from build123d import *

# Parameters (mm, degrees)
SKETCH1_R           = 1.3
SKETCH1_R_2         = 0.3
BOSS_EXTRUDE1_DEPTH = 1
SKETCH1_3_R         = 0.7625
BOSS_EXTRUDE2_DEPTH = 0.7
BOSS_EXTRUDE3_DEPTH = 0.6
BOSS_EXTRUDE4_DEPTH = 0.6
BOSS_EXTRUDE5_DEPTH = 0.2
SKETCH5_R           = 0.3
BOSS_EXTRUDE6_DEPTH = 0.2


with BuildPart() as part:
    # Sketch1 → Boss-Extrude1 (new, symmetric)
    with BuildSketch(Plane.XY):
        Circle(SKETCH1_R)
        Circle(SKETCH1_R_2, mode=Mode.SUBTRACT)
    extrude(amount=BOSS_EXTRUDE1_DEPTH, both=True)



with BuildPart() as body_2:
    # Sketch1_3 → Boss-Extrude2 (new, symmetric)
    with BuildSketch(Plane.XY):
        with Locations((3.98, -0.68)):
            Circle(SKETCH1_3_R)
    extrude(amount=BOSS_EXTRUDE2_DEPTH, both=True)


with BuildPart() as part_1:
    add(part.part)

    add(body_2.part)  # Boss-Extrude3 merges body 2
    # Sketch1_4 → Boss-Extrude3 (add, symmetric)
    with BuildSketch(Plane.XY):
        with BuildLine():
            ThreePointArc((3.432931907, -1.211152286), (3.227898468, -0.554502849), (3.635027175, 0))
            Line((3.635027175, 0), (1.875255399, 0.852756227))
            Line((1.875255399, 0.852756227), (0.329330809, 1.257593423))
            ThreePointArc((0.329330809, 1.257593423), (1.02910885, 0.794314153), (1.3, 0))
            ThreePointArc((1.3, 0), (1.158583747, -0.5896471), (0.765101997, -1.051008532))
            add(Edge.make_bspline(
                [(3.432931907, -1.211152286), (2.782696134, -0.927463912), (1.92467005, -0.895659575), (0.949941147, -0.916451296), (0.765101997, -1.051008532)],
                knots=[0, 0, 0, 0, 0.749641012, 1, 1, 1, 1], degree=3))
        make_face()
    extrude(amount=BOSS_EXTRUDE3_DEPTH, both=True)

    # Sketch1_5 → Boss-Extrude4 (add, symmetric)
    with BuildSketch(Plane.XY):
        with BuildLine():
            ThreePointArc((-1.295848634, -0.103809043), (-1.071749439, 0.735767042), (-0.368782161, 1.24659525))
            Line((-0.368782161, 1.24659525), (-1.982194984, 2.225541153))
            Line((-1.982194984, 2.225541153), (-3.468005165, 2.793231136))
            Line((-3.468005165, 2.793231136), (-3.852867925, 2.232623737))
            Line((-3.852867925, 2.232623737), (-2.789177956, 1.050055575))
            Line((-2.789177956, 1.050055575), (-1.295848634, -0.103809043))
        make_face()
    extrude(amount=BOSS_EXTRUDE4_DEPTH, both=True)



with BuildPart() as body_2_2:
    # Sketch2 → Revolve1 (revolve)
    with BuildSketch(Plane.XY, mode=Mode.PRIVATE) as revolve1_sk:
        with BuildLine():
            Line((-3.852867925, 2.232623737), (-3.445366179, 2.826208042))
            Line((-3.445366179, 2.826208042), (-3.771013124, 3.049768027))
            Line((-3.771013124, 3.049768027), (-4.831729785, 1.50468321))
            ThreePointArc((-4.831729785, 1.50468321), (-4.376188277, 1.556125039), (-4.362335635, 2.014352527))
            Line((-4.362335635, 2.014352527), (-3.852867925, 2.232623737))
        make_face()
    revolve(revolve1_sk.sketch.rotate(Axis((-3.771013124, 3.049768027, 0), (-0.5659746478395028, -0.8244226452511788, 0)), 180), axis=Axis((-3.771013124, 3.049768027, 0), (-0.5659746478395028, -0.8244226452511788, 0)))


with BuildPart() as part_2:
    add(part_1.part)

    add(body_2_2.part)  # Revolve2 merges body 2 2
    # Sketch3 → Revolve2 (revolve)
    with BuildSketch(Plane.XY):
        Polygon((-3.682752686, 3.178331919), (-4.291741407, 2.291253153), (-5.041966015, 2.806290082), (-4.432977294, 3.693368848), align=None)
    revolve(axis=Axis((-3.682752686, 3.178331919, 0), (-0.5659746478395036, -0.8244226452511781, 0)))

    # Sketch4 → Boss-Extrude5 (add, symmetric)
    with BuildSketch(Plane(origin=(0.303330803, 0.441844497, 0), x_dir=(0.824422645251178, -0.5659746478395038, 0), z_dir=(0.5659746478395038, 0.824422645251178, 0))):
        Polygon((-4.835, 0.75055535), (-5.485, 0.375277675), (-5.485, -0.375277675), (-4.835, -0.75055535), (-4.185, -0.375277675), (-4.185, 0.375277675), align=None)
    extrude(amount=BOSS_EXTRUDE5_DEPTH, both=True)

    # Sketch5 → Boss-Extrude6 (add, symmetric)
    with BuildSketch(Plane(origin=(0.416525733, 0.606729026, 0), x_dir=(0.8244226452511778, -0.5659746478395041, 0), z_dir=(0.565974647839504, 0.8244226452511777, 0))):
        with Locations(Location((-4.835, 0, 0), (0, 0, 180))):
            Circle(SKETCH5_R)
    extrude(amount=BOSS_EXTRUDE6_DEPTH, both=True)


solid = part_2.part
Read the model definition and answer for the solid it produces. Units are mm, in the model's axes. A direction names the side the tool comes from. Round coordinates to 2 decimals unless told otherwise and drop trailing zeros. Write each loop counter-clockwise with the first axis right and the second up, starting at its lowest first coordinate (ties: lowest second). Pieces come first, ordered by that corner, then holes. Notation, with made-up numbers: M -21,-8 L -6,-8 A24 cw -6,9 Z; hole C 26,-19.5 d11. An arc over 180 degrees is marked long. Use a Markdown table: item, result.
1) Straight lines are drawn through the part: line 1 along Y through (x, z) = (0, 0.35); line 2 along Y through (x, z) = (4, 0.6); line 3 along Z through (x, y) = (2, -0.65). For each, find the intervals that lie inside material, in ascending order. Write a range as [from, to].
Answers follow:
| item | result |
|---|---|
| line 1 | y = [-1.3, -0.3], [0.3, 1.3] |
| line 2 | y = [-1.44, 0.08] |
| line 3 | z = [-0.6, 0.6] |
2) The part is cut by section A-A (x = 0). Write down the section's boundary in (y, z), plus the area to 3 significant figures.
Answers follow:
| item | result |
|---|---|
| outline | M -1.3,-1 L -0.3,-1 L -0.3,1 L -1.3,1 Z; M 0.3,-1 L 1.3,-1 L 1.3,1 L 0.3,1 Z |
| area | 4.00 mm2 |
3) Flat-ended cylindrical pins translate along their axes: pin 1 (3 mm diameter, centred on x = -2, y = 0.5, fed in from -Z); pin 2 (0.8 mm diameter, centred on x = 4, y = -0.5, fed in from -Z); pin 3 (1.4 mm diameter, centred on x = -1.5, y = 1.5, fed in from +Z); pin 4 (0.5 mm diameter, centred on x = 4.5, y = -1, fed in from +Z). Find the tip coordinate at first contact, or state that the pin passes through.
Answers follow:
| item | result |
|---|---|
| pin 1 | stops at z = -1 |
| pin 2 | stops at z = -0.7 |
| pin 3 | stops at z = 0.6 |
| pin 4 | stops at z = 0.7 |
4) The part is cut by section C-C (z = 0.1). Give the number of separate pieces and of enclosed holes in the cut face, plus the area to 3 significant figures.
Answers follow:
| item | result |
|---|---|
| separate pieces | 2 |
| enclosed holes | 1 |
| area | 16.9 mm2 |
5) For a pull along Y with two mould halves and no side action, classify faces 4 (the flat face through (4, -1, -0.7)), 5 (the cylindrical face through (4.684, -0.972, 0.01)), 6 (the flat face through (-3.97, 2.07, 0.19)) as pulls with the +Y half, pulls with the -Y half, needs draft (parallel to the pull), parting line crosses it, or undercut.
Answers follow:
| item | result |
|---|---|
| face 4 | needs draft |
| face 5 | parting line crosses it |
| face 6 | undercut |
6) The part is cut by section B-B (y = 1.65). Write down the section's boundary in (x, z), plus the area to 3 significant figures.
Answers follow:
| item | result |
|---|---|
| outline | C -4.63,0 d0.64; M -3.33,-0.6 L -1.03,-0.6 L -1.03,0.6 L -3.33,0.6 Z |
| area | 3.07 mm2 |
7) The part is cut by section D-D (x = 3.98). Write down the section's boundary in (y, z), plus the area to 4 significant figures.
Answers follow:
| item | result |
|---|---|
| outline | M -1.44,-0.7 L 0.08,-0.7 L 0.08,0.7 L -1.44,0.7 Z |
| area | 2.135 mm2 |
8) A tool of negligible diameter and unlimited length cuts with its end or side. For faces 1 (the cylindrical face through (-0.28, -1.27, 0.01)), 2 (the flat face through (1.113, 1.052, -0.008)), 3 (the flat face through (4, -1, 0.7)), from which of +Z, -Z, +X, -X, +Y, -Y can it reach the whole face along a straight path? Write none if from no direction.
Answers follow:
| item | result |
|---|---|
| face 1 | none |
| face 2 | +Z, -Z, +X, +Y |
| face 3 | +Z, +X, +Y, -Y |
